```python
from build123d import *

# Parameters (mm, degrees)
BOSS_EXTRUDE1_DEPTH = 14.5
CUT_EXTRUDE1_DEPTH  = 12
SKETCH3_R           = 17.5
SKETCH3_R_2         = 12.7
BOSS_EXTRUDE2_DEPTH = 2
SKETCH4_R           = 5.5
CUT_EXTRUDE2_DEPTH  = 3.5
BOSS_EXTRUDE4_DEPTH = 12
SKETCH6_R           = 2.5
CUT_EXTRUDE4_DEPTH  = 10
SKETCH7_R           = 5.5
CUT_EXTRUDE5_DEPTH  = 10
FILLET1_R           = 0.5


with BuildPart() as part:
    # Sketch1 → Boss-Extrude1 (new body)
    with BuildSketch(Plane(origin=(0, 0, 0), x_dir=(1, 0, 0), z_dir=(0, 1, 0))):
        with BuildLine():
            Line((0, 45), (145, 45))
            ThreePointArc((145, 45), (190, 0), (145, -45))
            Line((145, -45), (0, -45))
            ThreePointArc((0, -45), (-45, 0), (0, 45))
        make_face()
    extrude(amount=BOSS_EXTRUDE1_DEPTH)

    # Sketch2 → Cut-Extrude1 (cut)
    with BuildSketch(Plane(origin=(0, 14.5, 0), x_dir=(1, 0, 0), z_dir=(0, 1, 0))):
        with BuildLine():
            Line((145, 42.5), (0, 42.5))
            ThreePointArc((0, 42.5), (-42.5, 0), (0, -42.5))
            Line((0, -42.5), (145, -42.5))
            ThreePointArc((145, -42.5), (187.5, 0), (145, 42.5))
        make_face()
    extrude(amount=-CUT_EXTRUDE1_DEPTH, mode=Mode.SUBTRACT)

    # Sketch3 → Boss-Extrude2 (add)
    with BuildSketch(Plane(origin=(0, 2.5, 0), x_dir=(1, 0, 0), z_dir=(0, 1, 0))):
        Circle(SKETCH3_R)
        Circle(SKETCH3_R_2, mode=Mode.SUBTRACT)
        with Locations((145, 0)):
            Circle(SKETCH3_R)
        with Locations((145, 0)):
            Circle(SKETCH3_R_2, mode=Mode.SUBTRACT)
    extrude(amount=BOSS_EXTRUDE2_DEPTH)

    # Sketch4 → Cut-Extrude2 (cut, through all)
    with BuildSketch(Plane(origin=(0, 2.5, 0), x_dir=(1, 0, 0), z_dir=(0, 1, 0))):
        with Locations((72.5, 0)):
            Circle(SKETCH4_R)
    extrude(amount=-CUT_EXTRUDE2_DEPTH, mode=Mode.SUBTRACT)

    # Sketch5 → Boss-Extrude4 (add)
    with BuildSketch(Plane(origin=(0, 2.5, 0), x_dir=(1, 0, 0), z_dir=(0, 1, 0))):
        with BuildLine():
            ThreePointArc((98.75, 42.5), (102.073598273, 40.823598273), (103.75, 37.5))
            ThreePointArc((103.75, 37.5), (108.75, 32.5), (113.75, 37.5))
            ThreePointArc((113.75, 37.5), (115.426401727, 40.823598273), (118.75, 42.5))
            Line((118.75, 42.5), (98.75, 42.5))
        make_face()
        with BuildLine():
            ThreePointArc((41.25, 37.5), (42.926401727, 40.823598273), (46.25, 42.5))
            Line((46.25, 42.5), (26.25, 42.5))
            ThreePointArc((26.25, 42.5), (29.573598273, 40.823598273), (31.25, 37.5))
            ThreePointArc((31.25, 37.5), (36.25, 32.5), (41.25, 37.5))
        make_face()
        with BuildLine():
            Line((98.75, -42.5), (118.75, -42.5))
            ThreePointArc((118.75, -42.5), (115.426401727, -40.823598273), (113.75, -37.5))
            ThreePointArc((113.75, -37.5), (108.75, -32.5), (103.75, -37.5))
            ThreePointArc((103.75, -37.5), (102.073598273, -40.823598273), (98.75, -42.5))
        make_face()
        with BuildLine():
            ThreePointArc((31.25, -37.5), (29.573598273, -40.823598273), (26.25, -42.5))
            Line((26.25, -42.5), (46.25, -42.5))
            ThreePointArc((46.25, -42.5), (42.926401727, -40.823598273), (41.25, -37.5))
            ThreePointArc((41.25, -37.5), (36.25, -32.5), (31.25, -37.5))
        make_face()
    extrude(amount=BOSS_EXTRUDE4_DEPTH)

    # Sketch6 → Cut-Extrude4 (cut)
    with BuildSketch(Plane(origin=(0, 14.5, 0), x_dir=(1, 0, 0), z_dir=(0, 1, 0))):
        with Locations((108.754596876, 37.512242845)):
            Circle(SKETCH6_R)
        with Locations((36.254596876, 37.512242845)):
            Circle(SKETCH6_R)
        with Locations((36.254596876, -37.512242845)):
            Circle(SKETCH6_R)
        with Locations((108.754596876, -37.512242845)):
            Circle(SKETCH6_R)
    extrude(amount=-CUT_EXTRUDE4_DEPTH, mode=Mode.SUBTRACT)

    # Sketch7 → Cut-Extrude5 (cut)
    with BuildSketch(Plane(origin=(0, 2.5, 0), x_dir=(1, 0, 0), z_dir=(0, 1, 0))):
        Circle(SKETCH7_R)
        with Locations((145, 0)):
            Circle(SKETCH7_R)
    extrude(amount=-CUT_EXTRUDE5_DEPTH, mode=Mode.SUBTRACT)

    # Fillet1
    fillet1_edges = [part.edges().sort_by_distance(p)[0] for p in [
        (-5.5, 0, 0),
        (139.5, 0, 0),
        (67, 0, 0),
        (72.5, 0, -45),
        (190, 0, 0),
        (72.5, 0, 45),
        (-45, 0, 0),
    ]]
    fillet(fillet1_edges, radius=FILLET1_R)


solid = part.part
```
Geometry check sheet. Reference: the model listing, model coordinates, mm. A direction names the side the tool comes from. Give positions to 0.01 mm unless a question says otherwise; leave off trailing zeros. Write each loop counter-clockwise with the first axis right and the second up, starting at its lowest first coordinate (ties: lowest second). Pieces come first, ordered by that corner, then holes. Notation, with made-up numbers: (77, 86.5) -> (82, 86.5) arc R18 ccw to (82, 100.5) -> close; hole circle Ø10 at (-13, -28.5). An arc over 180 degrees is marked (long way). One line per question, with ' | ' between items.
Item 1: Sectioned sample at C-C, the plane y = 12. Record the boundary of the cut face in (x, z).
Determined:
outline: (0, -45) -> (145, -45) arc R45 ccw to (145, 45) -> (0, 45) arc R45 ccw to start; hole (0, -42.5) -> (26.25, -42.5) arc R5.95 ccw to (31.25, -37.5) arc R5 cw to (41.25, -37.5) arc R5.95 ccw to (46.25, -42.5) -> (98.75, -42.5) arc R5.95 ccw to (103.75, -37.5) arc R5 cw to (113.75, -37.5) arc R5.95 ccw to (118.75, -42.5) -> (145, -42.5) arc R42.5 ccw to (145, 42.5) -> (118.75, 42.5) arc R5.95 ccw to (113.75, 37.5) arc R5 cw to (103.75, 37.5) arc R5.95 ccw to (98.75, 42.5) -> (46.25, 42.5) arc R5.95 ccw to (41.25, 37.5) arc R5 cw to (31.25, 37.5) arc R5.95 ccw to (26.25, 42.5) -> (0, 42.5) arc R42.5 ccw to start; hole circle Ø5 at (36.25, -37.51); hole circle Ø5 at (36.25, 37.51); hole circle Ø5 at (108.75, -37.51); hole circle Ø5 at (108.75, 37.51)
Item 2: Depth check by flat-ended pin: pin 1 (17.5 mm diameter, centred on x = 0.5, z = 2, fed in from +Y); pin 2 (10 mm diameter, centred on x = 123.5, z = 15, fed in from -Y); pin 3 (2.5 mm diameter, centred on x = 36.5, z = -38, fed in from +Y); pin 4 (3 mm diameter, centred on y = 5, z = -5, fed in from +X). Enter the tip coordinate at first touch or a pass-through.
Determined:
pin 1: y = 2.5 | pin 2: y = 0 | pin 3: y = 4.5 | pin 4: x = 189.86
Item 3: Sectioned sample at A-A, the plane x = 72.5. Record the boundary of the cut face in (y, z).
Determined:
outline: (0, -44.5) arc R0.5 ccw to (0.5, -45) -> (14.5, -45) -> (14.5, -42.5) -> (2.5, -42.5) -> (2.5, -5.5) -> (0.5, -5.5) arc R0.5 ccw to (0, -6) -> close; (0, 6) arc R0.5 ccw to (0.5, 5.5) -> (2.5, 5.5) -> (2.5, 42.5) -> (14.5, 42.5) -> (14.5, 45) -> (0.5, 45) arc R0.5 ccw to (0, 44.5) -> close
Item 4: Access from +Z, -Z, +X, -X, +Y, -Y to the whole of each face (thin tool, end or side, straight path). Record for faces 5 (the cylindrical face through (-1.19, 1.51, 5.37)), 6 (the cylindrical face through (-42.49, 8.58, -0.93)).
Determined:
face 5: +Y, -Y | face 6: +Y
Item 5: Draft check along X on faces 1 (the flat face through (13, 9, 42.5)), 2 (the cylindrical face through (189.99, 7.4, -0.99)), 3 (the flat face through (73, 14.5, -44)), 4 (the cylindrical face through (-13.887, 3.486, 10.648)). Enter one of: released by +X, released by -X, zero draft, split by the parting line, or undercut.
Determined:
face 1: undercut | face 2: released by +X | face 3: zero draft | face 4: undercut
Item 6: Scan lines: line 1 along X through (y, z) = (1.2, 0); line 2 along X through (y, z) = (3.3, 0); line 3 along X through (y, z) = (8, -1). Record each from-to range of solid material in increasing order.
Determined:
line 1: -45 to -5.5, 5.5 to 67, 78 to 139.5, 150.5 to 190 | line 2: -45 to -42.5, -17.5 to -12.7, 12.7 to 17.5, 127.5 to 132.3, 157.7 to 162.5, 187.5 to 190 | line 3: -44.99 to -42.49, 187.49 to 189.99
Item 7: Sectioned sample at B-B, the plane x = 36.25. Record the boundary of the cut face in (y, z).
Determined:
outline: (0, -44.5) arc R0.5 ccw to (0.5, -45) -> (14.5, -45) -> (14.5, -40.01) -> (4.5, -40.01) -> (4.5, -35.01) -> (14.5, -35.01) -> (14.5, -32.5) -> (2.5, -32.5) -> (2.5, 32.5) -> (14.5, 32.5) -> (14.5, 35.01) -> (4.5, 35.01) -> (4.5, 40.01) -> (14.5, 40.01) -> (14.5, 45) -> (0.5, 45) arc R0.5 ccw to (0, 44.5) -> close
